Solid Edge part; units mm, degrees
sketch "Sketch1" plane through (5.8669, 0, 0) normal (1, 0, 0) x (0, 1, 0)
  circle A0 centre (-8, 19.8987) radius 1.7
  circle A1 centre (8, 19.8987) radius 1.7
  line L0 (27.0472, 7.9) -> (27.0472, 12.9)
  line L1 (27.0472, 12.9) -> (11.5822, 12.9)
  line L2 (11.5822, 27.3385) -> (11.5822, 16.9)
  line L3 (4.1678, 27.3385) -> (11.5822, 27.3385)
  line L4 (4.1678, 16.9) -> (4.1678, 27.3385)
  line L5 (-4.5, 12.9) -> (4.1678, 12.9)
  line L6 (-4.5, 27.3385) -> (-4.5, 12.9)
  line L7 (-11.9144, 27.3385) -> (-4.5, 27.3385)
  line L8 (-11.9144, 20.2747) -> (-11.9144, 27.3385)
  line L9 (-11.9144, 20.2747) -> (-17.7524, 12.7936)
  line L10 (-17.7524, 12.7936) -> (-26.9528, 12.7936)
  line L11 (-26.9528, 12.7936) -> (-26.9528, 7.9)
  line L12 (-26.9528, 7.9) -> (27.0472, 7.9)
  arc A2 (11.5822, 12.9) -> (11.5822, 16.9) centre (11.5822, 14.9) cw
  arc A3 (4.1678, 16.9) -> (4.1678, 12.9) centre (4.1678, 14.9) cw
extrude "ExtrudedProtrusion_1" add sketch "Sketch1" along normal blind 10
sketch "Sketch2" plane through (10.8669, 19.3147, 12.9) normal (0, 0, 1) x (1, 0, 0)
  line L0 (1.5237, -20.1519) -> (2.4746, -19.3013)
  line L1 (1.5237, -18.3831) -> (2.4746, -19.3013)
  arc A0 (1.5237, -18.3831) -> (1.5237, -20.1519) centre (0.6696, -19.2675) ccw
  line L2 (1.8505, -41.2986) -> (3.1168, -42.5214)
  line L3 (3.1168, -42.5214) -> (1.8505, -43.7443)
  arc A1 (1.8505, -43.7443) -> (1.8505, -41.2986) centre (0.6696, -42.5214) cw
  line L4 (1.8505, 5.2093) -> (3.1168, 3.9865)
  line L5 (3.1168, 3.9865) -> (1.8505, 2.7636)
  arc A2 (1.8505, 2.7636) -> (1.8505, 5.2093) centre (0.6696, 3.9865) cw
extrude "Cutout1" cut sketch "Sketch2" against normal up to next
sketch "Sketch3" plane through (10.8669, -11.9144, 24.843) normal (0, -1, 0) x (0, 0, -1)
  line L0 (-0.2184, 1.1809) -> (1.0044, 2.4472)
  line L1 (1.0044, 2.4472) -> (2.2273, 1.1809)
  arc A0 (2.2273, 1.1809) -> (-0.2184, 1.1809) centre (1.0044, 0) cw
extrude "Cutout2" cut sketch "Sketch3" against normal through all
properties material "ABS Plastic, high impact"
The model under review builds one solid part; all positions refer to its coordinate system, in mm. A direction names the side the tool comes from. Give positions to 0.01 mm unless a question says otherwise; leave off trailing zeros. Write each loop counter-clockwise with the first axis right and the second up, starting at its lowest first coordinate (ties: lowest second). Pieces come first, ordered by that corner, then holes.
(1) Consider section B-B, the plane z = 9.5. Give the boundary of the cut face in (x, y), and give its area (3 significant figures).
(2) Consider section D-D, the plane x = 8.25. Give the boundary of the cut face in (y, z), and give its area (3 significant figures).
(3) Consider section A-A, the plane y = -8. Give the boundary of the cut face in (x, z), and give its area (3 significant figures).
(4) Consider section C-C, the plane z = 16. Give the boundary of the cut face in (x, y).
(5) Tool access review of faces 4 (the flat face through (12.69, 7.823, 23.236)), 5 (the flat face through (11, 4.168, 21)), 6 (the flat face through (11, -21, 12.794)), 7 (the flat face through (13.36, -23.81, 10.38)): name each direction out of +Z, -Z, +X, -X, +Y, -Y from which nothing blocks a thin tool from reaching the whole face with its end or side.
(6) For P1, Ø4.5, axis at x = 10.87, z = 23.84, coming from the -Y side; P2, Ø6, axis at y = 0.5, z = 18, coming from the -X side; P3, Ø4.5, axis at x = 10.5, y = 0, coming from the +Z side; P4, Ø1, axis at x = 9, z = 16.5, coming from the +Y side, all flat-tipped, find the tip position at first contact; note any pin that passes through.
(7) The part is to be moulded in two halves that separate along X. For faces 1 (the flat face through (12.67, 7.82, 24.46)), 2 (the cylindrical face through (10.308, 0.087, 10.435)), 3 (the cylindrical face through (10.797, 7.779, 18.213)), say which applies: released by +X, released by -X, zero draft, split by the parting line, or undercut.
(8) To check wall thickness, follow L1, parallel to Z at x = 10.75, y = -8; L2, parallel to Y at x = 13.25, z = 25; L3, parallel to Z at x = 12, y = 4.5. State the ranges of each line that lie inside material, in increasing order.
Returned:
1. outline: (5.87, -26.95) - (15.87, -26.95) - (15.87, 27.05) - (5.87, 27.05) - close; hole (12.39, -0.84) - (13.34, 0.01) - (12.39, 0.93) arc R1.23 ccw (long way) to start; hole (12.72, -24.43) - (13.98, -23.21) - (12.72, -21.98) arc R1.7 ccw (long way) to start; hole (12.72, 22.08) - (13.98, 23.3) - (12.72, 24.52) arc R1.7 ccw (long way) to start
1. area: 515 mm2
2. outline: (-26.95, 7.9) - (27.05, 7.9) - (27.05, 12.9) - (11.58, 12.9) arc R2 cw to (11.58, 16.9) - (11.58, 27.34) - (4.17, 27.34) - (4.17, 16.9) arc R2 cw to (4.17, 12.9) - (-4.5, 12.9) - (-4.5, 27.34) - (-11.91, 27.34) - (-11.91, 20.27) - (-17.75, 12.79) - (-26.95, 12.79) - close; hole circle Ø3.4 at (-8, 19.9); hole circle Ø3.4 at (8, 19.9)
2. area: 474 mm2
3. outline: (5.87, 7.9) - (15.87, 7.9) - (15.87, 18.2) - (5.87, 18.2) - close; (5.87, 21.6) - (15.87, 21.6) - (15.87, 27.34) - (5.87, 27.34) - close; hole (12.05, 22.62) - (13.31, 23.84) - (12.05, 25.06) arc R1.7 ccw (long way) to start
3. area: 151 mm2
4. outline: (5.87, -15.25) - (15.87, -15.25) - (15.87, -4.5) - (5.87, -4.5) - close; (5.87, 5.84) - (15.87, 5.84) - (15.87, 9.91) - (5.87, 9.91) - close
5. face 4: +Y, -Y
5. face 5: +Z, +X, -X
5. face 6: +Z, +X, -X, -Y
5. face 7: +Z, -Z
6. P1: stops at y = -11.91
6. P2: passes through
6. P3: stops at z = 12.9
6. P4: stops at y = 11.58
7. face 1: undercut
7. face 2: undercut
7. face 3: zero draft
8. L1: z = 7.9 to 18.2, 21.6 to 22.14, 25.53 to 27.34
8. L2: y = -11.91 to -4.5, 4.17 to 11.58
8. L3: z = 7.9 to 12.93, 16.87 to 22.57, 25.11 to 27.34
